Here's how the part is built. I have some questions about the finished solid (model axes, mm). A direction names the side the tool comes from. Round coordinates to 2 decimals unless told otherwise and drop trailing zeros. Order: outer loops, then holes, each group sorted by start corner. A loop starts at its lowest first (then second) coordinate and runs counter-clockwise, first axis right, second up. Notation, with made-up numbers: (86, 88) - (123, 88) arc R20 ccw to (123, 98) - close; hole circle Ø2 at (45, 62.25). An arc over 180 degrees is marked (long way). One line per item, written item: value.
from build123d import *

# Parameters (mm, degrees)
F0_W     = 31
F0_H     = 36
F1_DEPTH = 4
F2_R     = 6
F2_W     = 6
F2_H     = 29
F2_W_2   = 19.817460835
F2_H_2   = 20
F3_DEPTH = 25
F4_W     = 6
F4_H     = 7
F4_R     = 6
F5_DEPTH = 7
F6_DEPTH = 17
F8_DEPTH = 25
F9_F1_R  = 5
F9_F2_R  = 5
F10_R    = 3


# Not quite as in the source:
# - two fillets or chamfers of one size are made in one step


with BuildPart() as f1:
    # F0 (on Top) → F1 (new body)
    with BuildSketch(Plane.XY):
        with Locations((15.5, 18)):
            Rectangle(F0_W, F0_H)
    extrude(amount=F1_DEPTH)

    # F2 (on face) → F3 (cut)
    with BuildSketch(Plane.XY.offset(4)):
        with Locations((22, 28)):
            Circle(F2_R)
        with Locations((3, 21.5)):
            Rectangle(F2_W, F2_H)
        with Locations((21.0912695825, 10)):
            Rectangle(F2_W_2, F2_H_2)
    extrude(amount=-F3_DEPTH, mode=Mode.SUBTRACT)

    # F4 (on face) → F5 (join)
    with BuildSketch(Plane.XY.offset(4)):
        with Locations((3, 3.5)):
            Rectangle(F4_W, F4_H)
        Polygon((6, 36), (6, 7), (6, 0), (11.182539165, 0), (11.182539165, 20), (31, 20), (31, 36), align=None)
        with Locations((22, 28)):
            Circle(F4_R, mode=Mode.SUBTRACT)
    extrude(amount=F5_DEPTH)

    # F4 (on face) → F6 (join)
    with BuildSketch(Plane.XY.offset(4)):
        with Locations((3, 3.5)):
            Rectangle(F4_W, F4_H)
    extrude(amount=F6_DEPTH)

    # F7 (on face) → F8 (cut)
    with BuildSketch(Plane.XZ):
        with BuildLine():
            ThreePointArc((4.275, 3), (3.8063708499, 4.1313708499), (2.675, 4.6))
            ThreePointArc((2.675, 4.6), (1.5436291501, 1.8686291501), (4.275, 3))
        make_face()
        with BuildLine():
            ThreePointArc((4.275, 18), (1.5436291501, 19.1313708499), (2.675, 16.4))
            ThreePointArc((2.675, 16.4), (3.8063708499, 16.8686291501), (4.275, 18))
        make_face()
    extrude(amount=-F8_DEPTH, mode=Mode.SUBTRACT)

    # F9: fillet of radius 5 on 4 edges, made by hand

    # F9_f1
    f9_f1_edges = [f1.edges().sort_by_distance(p)[0] for p in [
        (6, 3.5, 11),
    ]]
    fillet(f9_f1_edges, radius=F9_F1_R)

    # F9_f2
    f9_f2_edges = [f1.edges().sort_by_distance(p)[0] for p in [
        (31, 36, 5.5),
        (6, 36, 5.5),
        (31, 20, 5.5),
    ]]
    fillet(f9_f2_edges, radius=F9_F2_R)

    # F10
    f10_edges = [f1.edges().sort_by_distance(p)[0] for p in [
        (11.182539, 20, 5.5),
    ]]
    fillet(f10_edges, radius=F10_R)


solid = f1.part
Q1. If we section it at C-C, the plane z = 2: Please give me the cut outline in (x, y).
Results list:
outline: (0, 0) - (1.43, 0) - (1.43, 7) - (0, 7) - close; (3.92, 0) - (11.18, 0) - (11.18, 17) arc R3 cw to (14.18, 20) - (26, 20) arc R5 ccw to (31, 25) - (31, 31) arc R5 ccw to (26, 36) - (11, 36) arc R5 ccw to (6, 31) - (6, 7) - (3.92, 7) - close; hole circle Ø12 at (22, 28)
Q2. If we section it at B-B, the plane y = 28: Please give me the cut outline in (x, z), then the cut area to 3 significant figures.
Results list:
outline: (6, 0) - (16, 0) - (16, 11) - (6, 11) - close; (28, 0) - (31, 0) - (31, 11) - (28, 11) - close
area: 143 mm²
Q3. Will these pins go through, and if not, where does the flat tip stop? pin 1 (3.5 mm diameter, centred on y = 9.5, z = 4, fed in from +X); pin 2 (3.5 mm diameter, centred on x = 20, z = 6.5, fed in from -Y); pin 3 (5.5 mm diameter, centred on y = 2.5, z = 18, fed in from +X).
Results list:
pin 1: x = 11.18
pin 2: y = 20
pin 3: x = 6.06
Q4. Which directions (+Z, -Z, +X, -X, +Y, -Y) give clear straight access to the entire face, cutting with the end or side of a thin tool? Please do faces 1 (the flat face through (6, 3, 18)), 2 (the flat face through (20, 20, 5)), 3 (the flat face through (6, 19, 5)), 4 (the flat face through (3, 4, 21)), 5 (the flat face through (19, 36, 5)).
Results list:
face 1: +Z, +X, +Y, -Y
face 2: +Z, -Z, +X, -Y
face 3: +Z, -Z, -X, +Y
face 4: +Z, +X, -X, +Y, -Y
face 5: +Z, -Z, +X, -X, +Y
Q5. If we section it at D-D, the plane y = 3: Please give me the cut outline in (x, z) (3 decimals), then the cut area to 3 significant figures.
Results list:
outline: (0, 0) - (11.183, 0) - (11.183, 11) - (11, 11) arc R5 cw to (6, 16) - (6, 21) - (0, 21) - close; hole circle Ø3.2 at (2.675, 3); hole circle Ø3.2 at (2.675, 18)
area: 172 mm²
Q6. If we section it at A-A, the plane x = 22: Please give me the cut outline in (y, z).
Results list:
outline: (20, 0) - (22, 0) - (22, 11) - (20, 11) - close; (34, 0) - (36, 0) - (36, 11) - (34, 11) - close
Q7. If I drill on line 1 along X through (y, z) = (3.5, 18) (3 decimals); line 2 along X through (y, z) = (2.25, 3) (3 decimals); line 3 along Z through (x, y) = (6.5, 20), over which ranges is the centre line in solid material (lowest first)?
Results list:
line 1: 0 to 1.075, 4.275 to 6
line 2: 0 to 1.075, 4.275 to 11.183
line 3: 0 to 11
